Part model, mm, in its own coordinate system. Face numbers are marked on the shaded views. Give positions to 0.01 mm unless a question says otherwise; leave off trailing zeros. Order: outer loops, then holes, each group sorted by start corner. A loop starts at its lowest first (then second) coordinate and runs counter-clockwise, first axis right, second up. Notation, with made-up numbers: M 76.5,82 L 117.5,82 A31 ccw 117.5,107 Z; hole C -37.5,5.5 d4. An arc over 180 degrees is marked long. Answer as a JSON object with one key per item and string values.
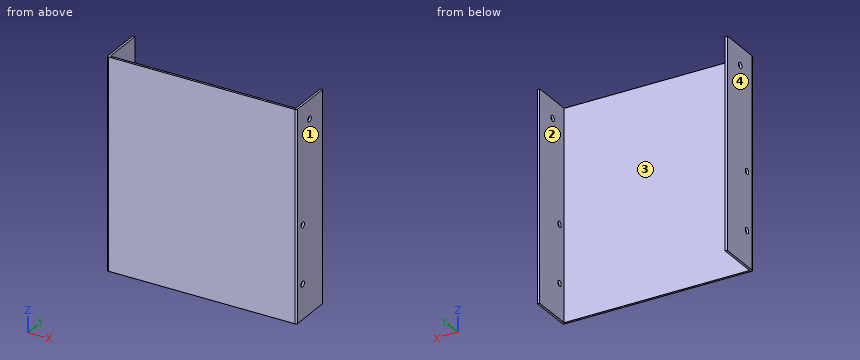
from build123d import *

# Parameters (mm, degrees)
SALIENTE_EXTRUIR1_DEPTH = 72.5
CROQUIS2_R              = 2
CORTAR_EXTRUIR1_DEPTH   = 145


with BuildPart() as part:
    # Croquis1 → Saliente-Extruir1 (new, symmetric)
    with BuildSketch(Plane.XY):
        with BuildLine():
            Line((-64.25, 14.5), (-64.25, -14))
            Line((-64.25, -14), (64.25, -14))
            Line((64.25, -14), (64.25, 14.5))
            Line((64.25, 14.5), (65.75, 14.5))
            Line((65.75, 14.5), (65.75, -14.5))
            ThreePointArc((65.75, -14.5), (65.457106781, -15.207106781), (64.75, -15.5))
            Line((64.75, -15.5), (-64.75, -15.5))
            ThreePointArc((-64.75, -15.5), (-65.457106781, -15.207106781), (-65.75, -14.5))
            Line((-65.75, -14.5), (-65.75, 14.5))
            Line((-65.75, 14.5), (-64.25, 14.5))
        make_face()
    extrude(amount=SALIENTE_EXTRUIR1_DEPTH, both=True)

    # Croquis2 → Cortar-Extruir1 (cut)
    with BuildSketch(Plane(origin=(65.75, 0, 0), x_dir=(0, 0, -1), z_dir=(1, 0, 0))):
        with Locations(Location((-59.5, -0.5, 0), (0, 0, 90))):
            Circle(CROQUIS2_R)
        with Locations(Location((8.5, -8.5, 0), (0, 0, 90))):
            Circle(CROQUIS2_R)
        with Locations(Location((48.5, -8.5, 0), (0, 0, 90))):
            Circle(CROQUIS2_R)
    extrude(amount=-CORTAR_EXTRUIR1_DEPTH, mode=Mode.SUBTRACT)


solid = part.part
1. Cut at A-A on y = 8.5. Give the cut face in (x, z), plus the area to 3 significant figures.
Worked answers:
{"outline": "M -65.75,-72.5 L -64.25,-72.5 L -64.25,72.5 L -65.75,72.5 Z; M 64.25,-72.5 L 65.75,-72.5 L 65.75,72.5 L 64.25,72.5 Z", "area": "435 mm^2"}
2. Two-plate mould, pull along X, no slides. Class the marked faces 1, 2, 3 and 4: +X half, -X half, draft (parallel to the pull), parting line (faces both ways), or undercut.
Worked answers:
{"face 1": "+X half", "face 2": "undercut", "face 3": "undercut", "face 4": "-X half"}
3. Pin check, flat tips, straight feed: P1, Ø5, axis at y = -8.5, z = -48.5, coming from the +X side; P2, Ø5, axis at x = -49.5, z = 9.5, coming from the +Y side. Stop position of each tip, or through.
Worked answers:
{"P1": "stops at x = 65.75", "P2": "stops at y = -14"}
4. Cut at D-D on y = -8.5. Give the cut face in (x, z).
Worked answers:
{"outline": "M -65.75,-72.5 L -64.25,-72.5 L -64.25,-50.5 L -65.75,-50.5 Z; M -65.75,-46.5 L -64.25,-46.5 L -64.25,-10.5 L -65.75,-10.5 Z; M -65.75,-6.5 L -64.25,-6.5 L -64.25,72.5 L -65.75,72.5 Z; M 64.25,-72.5 L 65.75,-72.5 L 65.75,-50.5 L 64.25,-50.5 Z; M 64.25,-46.5 L 65.75,-46.5 L 65.75,-10.5 L 64.25,-10.5 Z; M 64.25,-6.5 L 65.75,-6.5 L 65.75,72.5 L 64.25,72.5 Z"}
5. Cut at B-B on y = -0.5. Give the cut face in (x, z), plus the area to 3 significant figures.
Worked answers:
{"outline": "M -65.75,-72.5 L -64.25,-72.5 L -64.25,57.5 L -65.75,57.5 Z; M -65.75,61.5 L -64.25,61.5 L -64.25,72.5 L -65.75,72.5 Z; M 64.25,-72.5 L 65.75,-72.5 L 65.75,57.5 L 64.25,57.5 Z; M 64.25,61.5 L 65.75,61.5 L 65.75,72.5 L 64.25,72.5 Z", "area": "423 mm^2"}
6. Cut at C-C on z = -48.5. Give the cut face in (x, y), plus the area to 3 significant figures.
Worked answers:
{"outline": "M -65.75,-14.5 A1 ccw -64.75,-15.5 L 64.75,-15.5 A1 ccw 65.75,-14.5 L 65.75,-10.5 L 64.25,-10.5 L 64.25,-14 L -64.25,-14 L -64.25,-10.5 L -65.75,-10.5 Z; M -65.75,-6.5 L -64.25,-6.5 L -64.25,14.5 L -65.75,14.5 Z; M 64.25,-6.5 L 65.75,-6.5 L 65.75,14.5 L 64.25,14.5 Z", "area": "270 mm^2"}
7. Probe line 1 along Z through (x, y) = (-64.9, -8.5); line 2 along X through (y, z) = (-13, -26); line 3 along Y through (x, z) = (65, -8). List the from-to ranges inside material, lowest first.
Worked answers:
{"line 1": "z = -72.5 to -50.5, -46.5 to -10.5, -6.5 to 72.5", "line 2": "x = -65.75 to -64.25, 64.25 to 65.75", "line 3": "y = -15.47 to -10.44, -6.56 to 14.5"}
